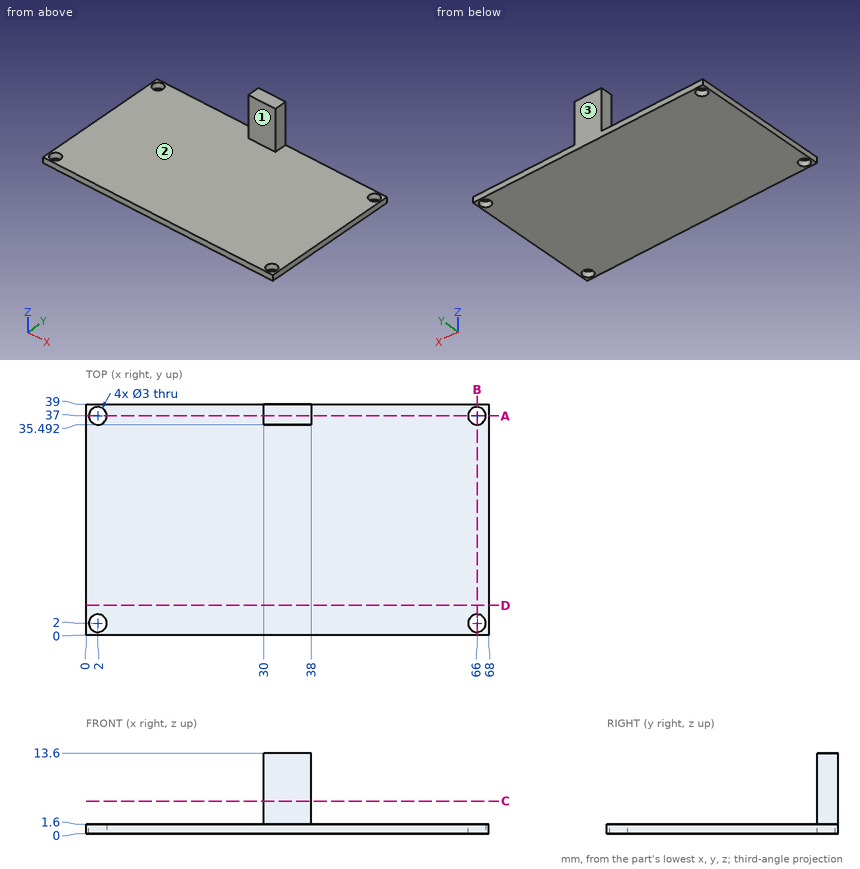
Part print with two shaded views. Sizes in mm from the minimum x, y, z corner. Coordinates: 2 decimals unless noted, no trailing zeros. Write each loop counter-clockwise with the first axis right and the second up, starting at its lowest first coordinate (ties: lowest second). Pieces come first, ordered by that corner, then holes. Notation, with made-up numbers: (0.25, 14) - (46.25, 14) arc R26 cw to (46.25, 49) - close; hole circle Ø7 at (6.5, 50.25). An arc over 180 degrees is marked (long way). Use a Markdown table: item, result. Add a question column.
Item 1: Drill centre lines: line 1 along Y through (x, z) = (2, 1); line 2 along Z through (x, y) = (10.5, 12.5); line 3 along Y through (x, z) = (35.5, 11.5). Where is each one in solid material? Low to high.
Item 2: Band-saw the part on B-B, the plane x = 66. Write the cut outline in (y, z), and give its area (3 significant figures).
Item 3: Two-plate mould, pull along Y, no slides. Class the marked faces 1, 2 and 3: pulls with the +Y half, pulls with the -Y half, needs draft (parallel to the pull), parting line crosses it, or undercut.
Item 4: Band-saw the part on D-D, the plane y = 5. Write the cut outline in (x, z).
Item 5: Band-saw the part on C-C, the plane z = 5.5. Write the cut outline in (x, y), and give its area (3 significant figures).
Item 6: Drop flat-ended pins along their axis: pin 1 (3 mm diameter, centred on y = 36.5, z = 5, fed in from +X); pin 2 (2 mm diameter, centred on x = 33.5, y = 21, fed in from +Z); pin 3 (4 mm diameter, centred on y = 38, z = 6, fed in from -X). Give the stop position or say it passes through.
Item 7: Band-saw the part on A-A, the plane y = 37. Write the cut outline in (x, z).
A:
| question | item | result |
|---|---|---|
| 1 | line 1 | y = 0 to 0.5, 3.5 to 35.5, 38.5 to 39 |
| 1 | line 2 | z = 0 to 1.6 |
| 1 | line 3 | y = 35.49 to 39 |
| 2 | outline | (0, 0) - (0.5, 0) - (0.5, 1.6) - (0, 1.6) - close; (3.5, 0) - (35.5, 0) - (35.5, 1.6) - (3.5, 1.6) - close; (38.5, 0) - (39, 0) - (39, 1.6) - (38.5, 1.6) - close |
| 2 | area | 52.8 mm² |
| 3 | face 1 | pulls with the -Y half |
| 3 | face 2 | needs draft |
| 3 | face 3 | pulls with the +Y half |
| 4 | outline | (0, 0) - (68, 0) - (68, 1.6) - (0, 1.6) - close |
| 5 | outline | (30, 35.49) - (38, 35.49) - (38, 39) - (30, 39) - close |
| 5 | area | 28.1 mm² |
| 6 | pin 1 | stops at x = 38 |
| 6 | pin 2 | stops at z = 1.6 |
| 6 | pin 3 | stops at x = 30 |
| 7 | outline | (0, 0) - (0.5, 0) - (0.5, 1.6) - (0, 1.6) - close; (3.5, 0) - (64.5, 0) - (64.5, 1.6) - (38, 1.6) - (38, 13.6) - (30, 13.6) - (30, 1.6) - (3.5, 1.6) - close; (67.5, 0) - (68, 0) - (68, 1.6) - (67.5, 1.6) - close |
